```python
from build123d import *

# Parameters (mm, degrees)
SKETCH1_R           = 1.5
BOTTOM_DEPTH        = 2
BOTTOM_2_DEPTH      = 2
BOTTOM_3_DEPTH      = 2
BOTTOM_4_DEPTH      = 2
WALLS_DEPTH         = 50
TOP_DEPTH           = 2
SKETCH4_R           = 1
SKETCH4_R_2         = 8.25
CUT_EXTRUDE2_DEPTH  = 2
SKETCH5_R           = 5
CUT_EXTRUDE3_DEPTH  = 2
SKETCH6_R           = 3
CUT_EXTRUDE4_DEPTH  = 2
SKETCH8_R           = 1.5
CUT_EXTRUDE5_DEPTH  = 2
BOSS_EXTRUDE5_DEPTH = 2
FILLET1_R           = 5
CUT_EXTRUDE6_DEPTH  = 10


with BuildPart() as part:
    # Sketch1 → Bottom (new body)
    with BuildSketch(Plane(origin=(0, 0, 0), x_dir=(1, 0, 0), z_dir=(0, 1, 0))):
        with BuildLine():
            ThreePointArc((-80, -45), (-71.213203436, -66.213203436), (-50, -75))
            Line((-50, -75), (-39.513159642, -75))
            Line((-39.513159642, -75), (-80, -34.513159642))
            Line((-80, -34.513159642), (-80, -45))
        make_face()
        with Locations(Location((-63.62, -59.64375, 0), (0, 0, 270))):
            Circle(SKETCH1_R, mode=Mode.SUBTRACT)
    extrude(amount=BOTTOM_DEPTH)



with BuildPart() as body_2:
    # Sketch1 → Bottom 2 (new body)
    with BuildSketch(Plane(origin=(0, 0, 0), x_dir=(1, 0, 0), z_dir=(0, 1, 0))):
        with BuildLine():
            Line((-80, 45), (-80, 34.513159642))
            Line((-80, 34.513159642), (-39.513159642, 75))
            Line((-39.513159642, 75), (-50, 75))
            ThreePointArc((-50, 75), (-71.213203436, 66.213203436), (-80, 45))
        make_face()
        with Locations(Location((-63.62, 59.64375, 0), (0, 0, 270))):
            Circle(SKETCH1_R, mode=Mode.SUBTRACT)
    extrude(amount=BOTTOM_2_DEPTH)


with BuildPart() as body_3:
    # Sketch1 → Bottom 3 (new body)
    with BuildSketch(Plane(origin=(0, 0, 0), x_dir=(1, 0, 0), z_dir=(0, 1, 0))):
        with BuildLine():
            Line((39.513159642, 75), (80, 34.513159642))
            Line((80, 34.513159642), (80, 45))
            ThreePointArc((80, 45), (71.213203436, 66.213203436), (50, 75))
            Line((50, 75), (39.513159642, 75))
        make_face()
        with Locations(Location((63.62, 59.64375, 0), (0, 0, 270))):
            Circle(SKETCH1_R, mode=Mode.SUBTRACT)
    extrude(amount=BOTTOM_3_DEPTH)


with BuildPart() as body_4:
    # Sketch1 → Bottom 4 (new body)
    with BuildSketch(Plane(origin=(0, 0, 0), x_dir=(1, 0, 0), z_dir=(0, 1, 0))):
        with BuildLine():
            Line((80, -34.513159642), (39.513159642, -75))
            Line((39.513159642, -75), (50, -75))
            ThreePointArc((50, -75), (71.213203436, -66.213203436), (80, -45))
            Line((80, -45), (80, -34.513159642))
        make_face()
        with Locations(Location((63.62, -59.64375, 0), (0, 0, 270))):
            Circle(SKETCH1_R, mode=Mode.SUBTRACT)
    extrude(amount=BOTTOM_4_DEPTH)


with BuildPart() as part_1:
    add(part.part)

    add(body_2.part)  # Walls merges body 2

    add(body_3.part)  # Walls merges body 3

    add(body_4.part)  # Walls merges body 4
    # Sketch2 → Walls (add)
    with BuildSketch(Plane(origin=(0, 2, 0), x_dir=(1, 0, 0), z_dir=(0, 1, 0))):
        with BuildLine():
            Line((50, 75), (-50, 75))
            ThreePointArc((-50, 75), (-71.213203436, 66.213203436), (-80, 45))
            Line((-80, 45), (-80, -45))
            ThreePointArc((-80, -45), (-71.213203436, -66.213203436), (-50, -75))
            Line((-50, -75), (50, -75))
            ThreePointArc((50, -75), (71.213203436, -66.213203436), (80, -45))
            Line((80, -45), (80, 45))
            ThreePointArc((80, 45), (71.213203436, 66.213203436), (50, 75))
        make_face()
        with BuildLine():
            Line((-48, -73), (48, -73))
            ThreePointArc((48, -73), (69.213203436, -64.213203436), (78, -43))
            Line((78, -43), (78, 43))
            ThreePointArc((78, 43), (69.213203436, 64.213203436), (48, 73))
            Line((48, 73), (-48, 73))
            ThreePointArc((-48, 73), (-69.213203436, 64.213203436), (-78, 43))
            Line((-78, 43), (-78, -43))
            ThreePointArc((-78, -43), (-69.213203436, -64.213203436), (-48, -73))
        make_face(mode=Mode.SUBTRACT)
    extrude(amount=WALLS_DEPTH)

    # Sketch3 → Top (add)
    with BuildSketch(Plane(origin=(0, 52, 0), x_dir=(1, 0, 0), z_dir=(0, 1, 0))):
        with BuildLine():
            Line((50, -75), (-50, -75))
            ThreePointArc((-50, -75), (-71.213203436, -66.213203436), (-80, -45))
            Line((-80, -45), (-80, 45))
            ThreePointArc((-80, 45), (-71.213203436, 66.213203436), (-50, 75))
            Line((-50, 75), (50, 75))
            ThreePointArc((50, 75), (71.213203436, 66.213203436), (80, 45))
            Line((80, 45), (80, -45))
            ThreePointArc((80, -45), (71.213203436, -66.213203436), (50, -75))
        make_face()
    extrude(amount=TOP_DEPTH)

    # Sketch4 → Cut-Extrude2 (cut)
    with BuildSketch(Plane.XY.offset(75)):
        with Locations((-20, 16.5)):
            Circle(SKETCH4_R)
        with Locations((-13.5, 24)):
            Circle(SKETCH4_R_2)
        with Locations(Location((-20, 31.5, 0), (0, 0, 180))):
            Circle(SKETCH4_R)
        with Locations((20, 16.5)):
            Circle(SKETCH4_R)
        with Locations((13.5, 24)):
            Circle(SKETCH4_R_2)
        with Locations((20, 31.5)):
            Circle(SKETCH4_R)
    extrude(amount=-CUT_EXTRUDE2_DEPTH, mode=Mode.SUBTRACT)

    # Sketch5 → Cut-Extrude3 (cut)
    with BuildSketch(Plane.XY.offset(75)):
        with Locations((-40, 28)):
            Circle(SKETCH5_R)
        with Locations((40, 28)):
            Circle(SKETCH5_R)
    extrude(amount=-CUT_EXTRUDE3_DEPTH, mode=Mode.SUBTRACT)

    # Sketch6 → Cut-Extrude4 (cut)
    with BuildSketch(Plane(origin=(0, 0, -75), x_dir=(-1, 0, 0), z_dir=(0, 0, -1))):
        with Locations((-40, 34)):
            Circle(SKETCH6_R)
    extrude(amount=-CUT_EXTRUDE4_DEPTH, mode=Mode.SUBTRACT)

    # Sketch8 → Cut-Extrude5 (cut)
    with BuildSketch(Plane(origin=(0, 54, 0), x_dir=(1, 0, 0), z_dir=(0, 1, 0))):
        with Locations(Location((-65, 0, 0), (0, 0, 270))):
            Circle(SKETCH8_R)
        with Locations(Location((65, 0, 0), (0, 0, 90))):
            Circle(SKETCH8_R)
    extrude(amount=-CUT_EXTRUDE5_DEPTH, mode=Mode.SUBTRACT)

    # Sketch9 → Boss-Extrude5 (add)
    with BuildSketch(Plane.XZ.offset(-2)):
        Polygon((-80, 34.513159642), (-78, 36.513159642), (-78, -36.513159642), (-80, -34.513159642), align=None)
        Polygon((-39.513159642, 75), (-41.513159642, 73), (41.513159642, 73), (39.745521731, 74.76763791), (39.513159642, 75), align=None)
        Polygon((78, -36.513159642), (80, -34.513159642), (80, 34.513159642), (78, 36.513159642), align=None)
        Polygon((39.745521731, -74.76763791), (39.513159642, -75), (-39.513159642, -75), (-41.513159642, -73), (41.513159642, -73), align=None)
    extrude(amount=BOSS_EXTRUDE5_DEPTH)

    # Fillet1
    fillet1_edges = [part_1.edges().sort_by_distance(p)[0] for p in [
        (-71.213203436, 54, 66.213203436),
        (0, 54, 75),
        (71.213203436, 54, 66.213203436),
        (80, 54, 0),
        (71.213203436, 54, -66.213203436),
        (0, 54, -75),
        (-71.213203436, 54, -66.213203436),
        (-80, 54, 0),
    ]]
    fillet(fillet1_edges, radius=FILLET1_R)

    # Sketch10 → Cut-Extrude6 (cut)
    with BuildSketch(Plane(origin=(0, 0, -75), x_dir=(-1, 0, 0), z_dir=(0, 0, -1))):
        with BuildLine():
            Line((6.5, 5), (-6.5, 5))
            ThreePointArc((-6.5, 5), (-7.207106781, 5.292893219), (-7.5, 6))
            Line((-7.5, 6), (-7.5, 12))
            ThreePointArc((-7.5, 12), (-7.207106781, 12.707106781), (-6.5, 13))
            Line((-6.5, 13), (6.5, 13))
            ThreePointArc((6.5, 13), (7.207106781, 12.707106781), (7.5, 12))
            Line((7.5, 12), (7.5, 6))
            ThreePointArc((7.5, 6), (7.207106781, 5.292893219), (6.5, 5))
        make_face()
    extrude(amount=-CUT_EXTRUDE6_DEPTH, mode=Mode.SUBTRACT)


solid = part_1.part
```
Work out the finished part from the listing and answer in its coordinate system (mm). A direction names the side the tool comes from. Give positions to 0.01 mm unless a question says otherwise; leave off trailing zeros. Order: outer loops, then holes, each group sorted by start corner. A loop starts at its lowest first (then second) coordinate and runs counter-clockwise, first axis right, second up. Notation, with made-up numbers: M -6,29.25 L 16,29.25 A7 cw 16,35.25 Z; hole C 31,-20 d9. An arc over 180 degrees is marked long. Return JSON: item names as keys, results as strings.
1) Straight lines are drawn through the part: line 1 along Z through (x, y) = (21, 11.5); line 2 along Y through (x, z) = (-40, 74); line 3 along X through (y, z) = (13, -31). For each, find the intervals that lie inside material, in ascending order. Write a range as [from, to].
Resolved:
{"line 1": "[-75, -73], [73, 75]", "line 2": "[0, 23], [33, 52]", "line 3": "[-80, -78], [78, 80]"}
2) Each of these flat-tipped pins is pushed along its axis until it touches: pin 1 (0.6 mm diameter, centred on x = -2.5, z = -74.5, fed in from +Y); pin 2 (5 mm diameter, centred on y = 14, z = -46, fed in from -X); pin 3 (6 mm diameter, centred on y = 35, z = 56, fed in from +X); pin 4 (6 mm diameter, centred on x = -58, y = 15, fed in from -Z). Where does it stop, or does it pass through?
Resolved:
{"pin 1": "y = 51.71", "pin 2": "x = -80", "pin 3": "x = 78.91", "pin 4": "z = -74.58"}
3) Section B-B, the plane x = 16.5 is taken. Write down the section's boundary in (y, z).
Resolved:
{"outline": "M 0,-75 L 49,-75 A5 ccw 54,-70 L 54,70 A5 ccw 49,75 L 31.69,75 L 31.69,73 L 52,73 L 52,-73 L 0,-73 Z; M 0,73 L 16.31,73 L 16.31,75 L 0,75 Z"}
4) A tool of negligible diameter and unlimited length cuts with its end or side. For faces 4 (the flat face through (-60.012, 0.986, -54.501)), 5 (the cylindrical face through (42.21, 36.03, -74.01)), 6 (the flat face through (64, 2, 57)), from which of +Z, -Z, +X, -X, +Y, -Y can it reach the whole face along a straight path? Write none if from no direction.
Resolved:
{"face 4": "-Y", "face 5": "-Z", "face 6": "none"}
5) Section A-A, the plane y = 39.5 is taken. Write down the section's boundary in (x, z), plus the area to 3 significant figures.
Resolved:
{"outline": "M -80,-45 A30 ccw -50,-75 L 50,-75 A30 ccw 80,-45 L 80,45 A30 ccw 50,75 L -50,75 A30 ccw -80,45 Z; hole M -78,-43 A30 ccw -48,-73 L 48,-73 A30 ccw 78,-43 L 78,43 A30 ccw 48,73 L -48,73 A30 ccw -78,43 Z", "area": "1,220 mm^2"}
6) For a pull along X with two mould halves and no side action, classify faces 1 (the cylindrical face through (-45, 28, 74)), 2 (the flat face through (54, 0, 61)), 3 (the flat face through (80, 24, -1)) as +X half, -X half, draft (parallel to the pull), parting line (faces both ways), or undercut.
Resolved:
{"face 1": "undercut", "face 2": "draft", "face 3": "+X half"}
7) Section D-D, the plane x = -27 is taken. Write down the section's boundary in (y, z).
Resolved:
{"outline": "M 0,-75 L 49,-75 A5 ccw 54,-70 L 54,70 A5 ccw 49,75 L 0,75 L 0,73 L 52,73 L 52,-73 L 0,-73 Z"}
8) Section C-C, the plane z = 13 is taken. Write down the section's boundary in (x, y).
Resolved:
{"outline": "M -80,0 L -78,0 L -78,52 L 78,52 L 78,0 L 80,0 L 80,49 A5 ccw 75,54 L -75,54 A5 ccw -80,49 Z"}
